Print and shaded views of the part. All mm, measured from the part's lowest x, y and z. A direction names the side the tool comes from. Round coordinates to 2 decimals unless told otherwise and drop trailing zeros. Loops run counter-clockwise (first coordinate to the right, second up) from the corner with the lowest first, then second, coordinate; pieces in that order, holes last. Notation, with made-up numbers: (45.25, 53) -> (87.25, 53) arc R16 ccw to (87.25, 69) -> close; hole circle Ø3 at (30, 37.25). An arc over 180 degrees is marked (long way). Answer as CSV lines item,"result".
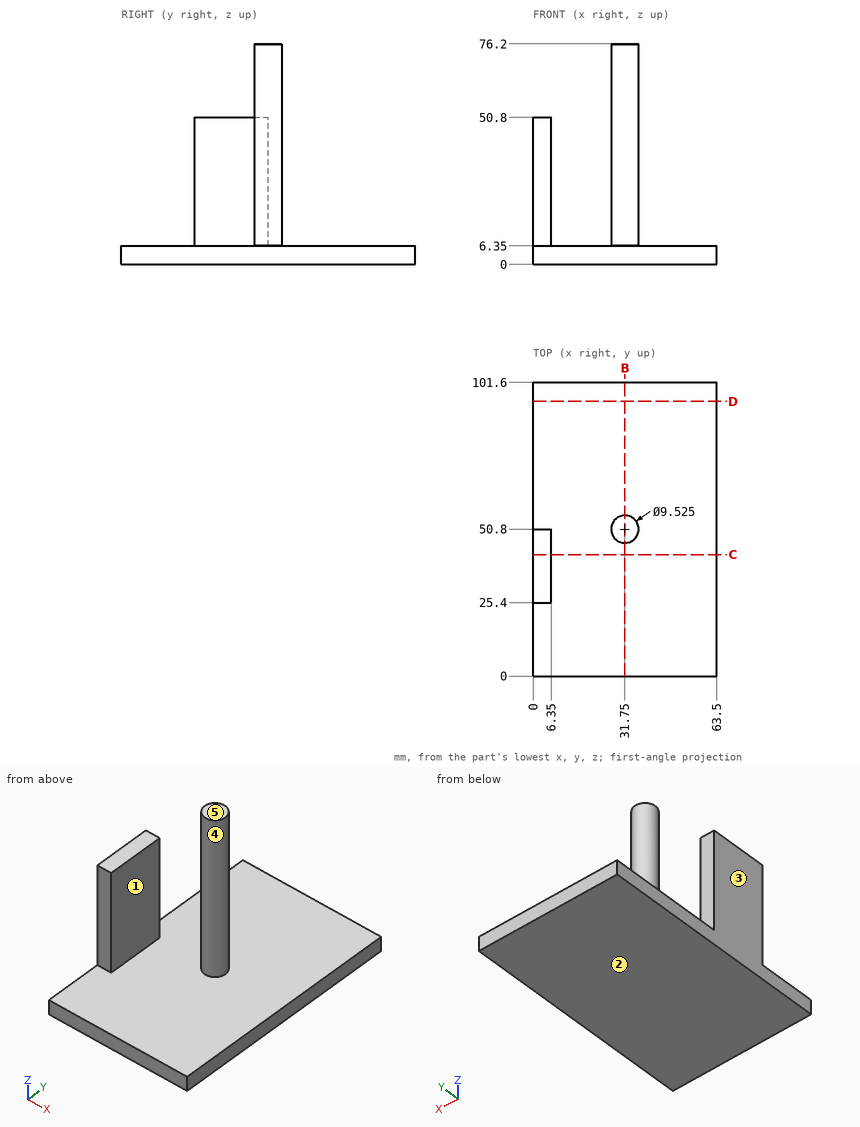
Q1. Slice it at D-D, the plane y = 95. Give the cut face in (x, z), and give its area (3 significant figures).
Results:
outline,"(0, 0) -> (63.5, 0) -> (63.5, 6.35) -> (0, 6.35) -> close"
area,"403 mm2"
Q2. Probe L1, parallel to Z at x = 49.5, y = 17; L2, parallel to X at y = 47.5, z = 23; L3, parallel to X at y = 50, z = 18. List the from-to ranges inside material, lowest first. Write a range as [from, to].
Results:
L1,"[0, 6.35]"
L2,"[0, 6.35], [28.32, 35.18]"
L3,"[0, 6.35], [27.06, 36.44]"
Q3. Drop flat-ended pins along their axis: pin 1 Ø3 at (x, z) = (2, 22.5) entering from -Y; pin 2 Ø7 at (x, y) = (3.5, 35.5) entering from +Z; pin 3 Ø5 at (x, z) = (29.5, 36.5) entering from +Y; pin 4 Ø5 at (y, z) = (59, 44.5) entering from +X. Give the stop position or say it passes through.
Results:
pin 1,"y = 25.4"
pin 2,"z = 50.8"
pin 3,"y = 55.56"
pin 4,"through"
Q4. Two-plate mould, pull along X, no slides. Class the marked faces 3, 4 and 5: pulls with the +X half, pulls with the -X half, needs draft (parallel to the pull), parting line crosses it, or undercut.
Results:
face 3,"pulls with the -X half"
face 4,"undercut"
face 5,"needs draft"
Q5. Slice it at C-C, the plane y = 42. Give the cut face in (x, z), and give its area (3 significant figures).
Results:
outline,"(0, 0) -> (63.5, 0) -> (63.5, 6.35) -> (6.35, 6.35) -> (6.35, 50.8) -> (0, 50.8) -> close"
area,"685 mm2"
Q6. Tool access for the marked faces 1 and 2: list every direction of +Z, -Z, +X, -X, +Y, -Y with a clear straight run to the whole face (end or side of a thin tool).
Results:
face 1,"+Z, +Y, -Y"
face 2,"-Z, +X, -X, +Y, -Y"
Q7. Slice it at B-B, the plane x = 31.75. Give the cut face in (y, z).
Results:
outline,"(0, 0) -> (101.6, 0) -> (101.6, 6.35) -> (55.56, 6.35) -> (55.56, 76.2) -> (46.04, 76.2) -> (46.04, 6.35) -> (0, 6.35) -> close"
